```python
from build123d import *

# Parameters (mm, degrees)
BOSS_EXTRUDE1_DEPTH = 6.35
M3_TAP_HOLES_REACH  = 72.995
SKETCH2_R           = 1.25


with BuildPart() as part:
    # Sketch1 → Boss-Extrude1 (new body)
    with BuildSketch(Plane(origin=(0, 0, 0), x_dir=(1, 0, 0), z_dir=(0, 1, 0))):
        with BuildLine():
            ThreePointArc((50, 0), (44.781853835, 22.239279825), (30.216577315, 39.83664714))
            Line((30.216577315, 39.83664714), (28.403582676, 37.446448312))
            ThreePointArc((28.403582676, 37.446448312), (42.094942605, 20.904923035), (47, 0))
            ThreePointArc((47, 0), (42.094942605, -20.904923035), (28.403582676, -37.446448312))
            Line((28.403582676, -37.446448312), (30.216577315, -39.83664714))
            ThreePointArc((30.216577315, -39.83664714), (44.781853835, -22.239279825), (50, 0))
        make_face()
        with BuildLine():
            ThreePointArc((43, 0), (38.512394298, 19.125780649), (25.986256491, 34.259516541))
            Line((25.986256491, 34.259516541), (24.173261852, 31.869317712))
            ThreePointArc((24.173261852, 31.869317712), (35.825483068, 17.79142386), (40, 0))
            ThreePointArc((40, 0), (35.825483068, -17.79142386), (24.173261852, -31.869317712))
            Line((24.173261852, -31.869317712), (25.986256491, -34.259516541))
            ThreePointArc((25.986256491, -34.259516541), (38.512394298, -19.125780649), (43, 0))
        make_face()
        with BuildLine():
            ThreePointArc((16.6764834, -39.634516541), (21.5, -37.239092363), (25.986256491, -34.259516541))
            Line((25.986256491, -34.259516541), (24.173261852, -31.869317712))
            ThreePointArc((24.173261852, -31.869317712), (20, -34.641016151), (15.513007814, -36.869317712))
            Line((15.513007814, -36.869317712), (16.6764834, -39.634516541))
        make_face()
        with BuildLine():
            ThreePointArc((18.227784182, -43.321448312), (23.5, -40.703193978), (28.403582676, -37.446448312))
            Line((28.403582676, -37.446448312), (25.986256491, -34.259516541))
            ThreePointArc((25.986256491, -34.259516541), (21.5, -37.239092363), (16.6764834, -39.634516541))
            Line((16.6764834, -39.634516541), (18.227784182, -43.321448312))
        make_face()
        with BuildLine():
            ThreePointArc((19.391259768, -46.08664714), (25, -43.301270189), (30.216577315, -39.83664714))
            Line((30.216577315, -39.83664714), (28.403582676, -37.446448312))
            ThreePointArc((28.403582676, -37.446448312), (23.5, -40.703193978), (18.227784182, -43.321448312))
            Line((18.227784182, -43.321448312), (19.391259768, -46.08664714))
        make_face()
        with BuildLine():
            ThreePointArc((-49.607837082, -6.25), (-25, -43.301270189), (19.391259768, -46.08664714))
            Line((19.391259768, -46.08664714), (18.227784182, -43.321448312))
            ThreePointArc((18.227784182, -43.321448312), (-23.5, -40.703193978), (-46.631366858, -5.875))
            Line((-46.631366858, -5.875), (-49.607837082, -6.25))
        make_face()
        with BuildLine():
            ThreePointArc((-42.662739891, -5.375), (-21.5, -37.239092363), (16.6764834, -39.634516541))
            Line((16.6764834, -39.634516541), (15.513007814, -36.869317712))
            ThreePointArc((15.513007814, -36.869317712), (-20, -34.641016151), (-39.686269666, -5))
            Line((-39.686269666, -5), (-42.662739891, -5.375))
        make_face()
        with BuildLine():
            Line((-39.686269666, 5), (-42.662739891, 5.375))
            ThreePointArc((-42.662739891, 5.375), (-43, 0), (-42.662739891, -5.375))
            Line((-42.662739891, -5.375), (-39.686269666, -5))
            ThreePointArc((-39.686269666, -5), (-40, 0), (-39.686269666, 5))
        make_face()
        with BuildLine():
            Line((-42.662739891, 5.375), (-46.631366858, 5.875))
            ThreePointArc((-46.631366858, 5.875), (-47, 0), (-46.631366858, -5.875))
            Line((-46.631366858, -5.875), (-42.662739891, -5.375))
            ThreePointArc((-42.662739891, -5.375), (-43, 0), (-42.662739891, 5.375))
        make_face()
        with BuildLine():
            Line((-46.631366858, 5.875), (-49.607837082, 6.25))
            ThreePointArc((-49.607837082, 6.25), (-50, 0), (-49.607837082, -6.25))
            Line((-49.607837082, -6.25), (-46.631366858, -5.875))
            ThreePointArc((-46.631366858, -5.875), (-47, 0), (-46.631366858, 5.875))
        make_face()
        with BuildLine():
            Line((18.227784182, 43.321448312), (19.391259768, 46.08664714))
            ThreePointArc((19.391259768, 46.08664714), (-25, 43.301270189), (-49.607837082, 6.25))
            Line((-49.607837082, 6.25), (-46.631366858, 5.875))
            ThreePointArc((-46.631366858, 5.875), (-23.5, 40.703193978), (18.227784182, 43.321448312))
        make_face()
        with BuildLine():
            Line((15.513007814, 36.869317712), (16.6764834, 39.634516541))
            ThreePointArc((16.6764834, 39.634516541), (-21.5, 37.239092363), (-42.662739891, 5.375))
            Line((-42.662739891, 5.375), (-39.686269666, 5))
            ThreePointArc((-39.686269666, 5), (-20, 34.641016151), (15.513007814, 36.869317712))
        make_face()
        with BuildLine():
            Line((24.173261852, 31.869317712), (25.986256491, 34.259516541))
            ThreePointArc((25.986256491, 34.259516541), (21.5, 37.239092363), (16.6764834, 39.634516541))
            Line((16.6764834, 39.634516541), (15.513007814, 36.869317712))
            ThreePointArc((15.513007814, 36.869317712), (20, 34.641016151), (24.173261852, 31.869317712))
        make_face()
        with BuildLine():
            Line((25.986256491, 34.259516541), (28.403582676, 37.446448312))
            ThreePointArc((28.403582676, 37.446448312), (23.5, 40.703193978), (18.227784182, 43.321448312))
            Line((18.227784182, 43.321448312), (16.6764834, 39.634516541))
            ThreePointArc((16.6764834, 39.634516541), (21.5, 37.239092363), (25.986256491, 34.259516541))
        make_face()
        with BuildLine():
            Line((28.403582676, 37.446448312), (30.216577315, 39.83664714))
            ThreePointArc((30.216577315, 39.83664714), (25, 43.301270189), (19.391259768, 46.08664714))
            Line((19.391259768, 46.08664714), (18.227784182, 43.321448312))
            ThreePointArc((18.227784182, 43.321448312), (23.5, 40.703193978), (28.403582676, 37.446448312))
        make_face()
    extrude(amount=BOSS_EXTRUDE1_DEPTH)

    # Sketch2 → M3-tap-holes (cut, up to next)
    with BuildSketch(Plane(origin=(0, 6.35, 0), x_dir=(1, 0, 0), z_dir=(0, 1, 0)), mode=Mode.PRIVATE) as m3_tap_holes_sk1:
        with Locations(Location((-45, 0, 0), (0, 0, 270))):
            Circle(SKETCH2_R)
    m3_tap_holes_tool1 = extrude(m3_tap_holes_sk1.sketch, amount=-M3_TAP_HOLES_REACH, mode=Mode.PRIVATE) & part.part
    # Sketch2 → M3-tap-holes (cut, up to next)
    with BuildSketch(Plane(origin=(0, 6.35, 0), x_dir=(1, 0, 0), z_dir=(0, 1, 0)), mode=Mode.PRIVATE) as m3_tap_holes_sk2:
        with Locations(Location((22.5, -38.97114317, 0), (0, 0, 270))):
            Circle(SKETCH2_R)
    m3_tap_holes_tool2 = extrude(m3_tap_holes_sk2.sketch, amount=-M3_TAP_HOLES_REACH, mode=Mode.PRIVATE) & part.part
    # Sketch2 → M3-tap-holes (cut, up to next)
    with BuildSketch(Plane(origin=(0, 6.35, 0), x_dir=(1, 0, 0), z_dir=(0, 1, 0)), mode=Mode.PRIVATE) as m3_tap_holes_sk3:
        with Locations(Location((22.5, 38.97114317, 0), (0, 0, 270))):
            Circle(SKETCH2_R)
    m3_tap_holes_tool3 = extrude(m3_tap_holes_sk3.sketch, amount=-M3_TAP_HOLES_REACH, mode=Mode.PRIVATE) & part.part
    add(m3_tap_holes_tool1.solids().sort_by_distance((-45, 6.35, 0))[0], mode=Mode.SUBTRACT)
    add(m3_tap_holes_tool2.solids().sort_by_distance((22.5, 6.35, 38.971143))[0], mode=Mode.SUBTRACT)
    add(m3_tap_holes_tool3.solids().sort_by_distance((22.5, 6.35, -38.971143))[0], mode=Mode.SUBTRACT)


solid = part.part
```
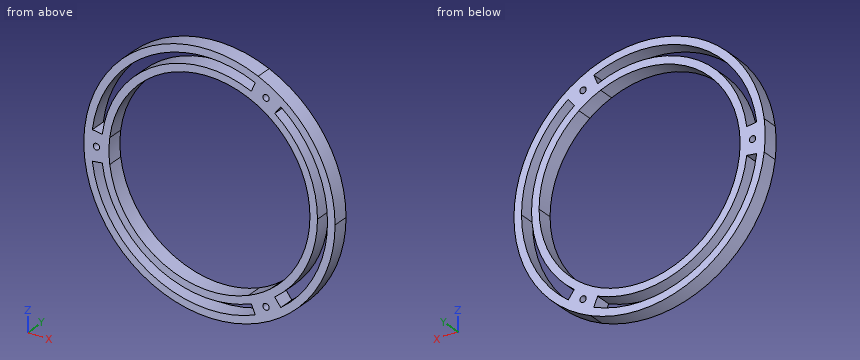
The listing builds one solid part. Answer for the finished solid, in the listing's coordinates (mm). Coordinates: 2 decimals unless noted, no trailing zeros. Loops run counter-clockwise (first coordinate to the right, second up) from the corner with the lowest first, then second, coordinate; pieces in that order, holes last. Notation, with made-up numbers: (47.25, 19) -> (68.25, 19) arc R20 cw to (68.25, 34) -> close; hole circle Ø1 at (36.5, -38.5). An arc over 180 degrees is marked (long way). Use one line per item in the form item = value. Start each with the question number.
Item 1: The part is cut by section B-B on y = 1.25. Determine the outline of the cut face in (x, z) (3 decimals).
Item 2: Consider L1, parallel to X at y = 4.5, z = 11 (3 decimals); L2, parallel to X at y = 3.75, z = -9. Determine where each line is inside the solid, lowest interval first. Write a range as [from, to].
Item 3: Flat-ended cylindrical pins translate along their axes: pin 1 Ø12 at (x, z) = (-36.5, 4) entering from +Y; pin 2 Ø10 at (x, z) = (18.5, -29.5) entering from -Y; pin 3 Ø2 at (x, y) = (4.5, 1) entering from +Z. Find the tip coordinate at first contact, or state that the pin passes through.
Item 4: The part is cut by section C-C on z = 13.5. Determine the outline of the cut face in (x, y), then the cut area to 3 significant figures.
Item 5: The part is cut by section A-A on x = 35. Determine the outline of the cut face in (y, z).
Answer key:
q1.outline = circle Ø100 at (0, 0); hole (-46.631, -5.875) arc R47 ccw to (18.228, -43.321) -> (16.676, -39.635) arc R43 cw to (-42.663, -5.375) -> close; hole (-46.631, 5.875) -> (-42.663, 5.375) arc R43 cw to (16.676, 39.635) -> (18.228, 43.321) arc R47 ccw to start; hole circle Ø2.5 at (-45, 0); hole circle Ø80 at (0, 0); hole circle Ø2.5 at (22.5, -38.971); hole circle Ø2.5 at (22.5, 38.971); hole (25.986, -34.26) -> (28.404, -37.446) arc R47 ccw to (28.404, 37.446) -> (25.986, 34.26) arc R43 cw to start
q2.L1 = [-48.775, -45.695], [-41.569, -38.458], [38.458, 41.569], [45.695, 48.775]
q2.L2 = [-49.18, -46.13], [-42.05, -38.97], [38.97, 42.05], [46.13, 49.18]
q3.pin_1 = 6.35
q3.pin_2 = through
q3.pin_3 = 49.88
q4.outline = (-48.14, 0) -> (-45.02, 0) -> (-45.02, 6.35) -> (-48.14, 6.35) -> close; (-40.83, 0) -> (-37.65, 0) -> (-37.65, 6.35) -> (-40.83, 6.35) -> close; (37.65, 0) -> (40.83, 0) -> (40.83, 6.35) -> (37.65, 6.35) -> close; (45.02, 0) -> (48.14, 0) -> (48.14, 6.35) -> (45.02, 6.35) -> close
q4.area = 80.0 mm2
q5.outline = (0, -35.71) -> (6.35, -35.71) -> (6.35, -31.37) -> (0, -31.37) -> close; (0, -24.98) -> (6.35, -24.98) -> (6.35, -19.36) -> (0, -19.36) -> close; (0, 19.36) -> (6.35, 19.36) -> (6.35, 24.98) -> (0, 24.98) -> close; (0, 31.37) -> (6.35, 31.37) -> (6.35, 35.71) -> (0, 35.71) -> close
